Build history of the part. All positions in model axes, mm. A direction names the side the tool comes from. Round coordinates to 2 decimals unless told otherwise and drop trailing zeros. Write each loop counter-clockwise with the first axis right and the second up, starting at its lowest first coordinate (ties: lowest second). Pieces come first, ordered by that corner, then holes. Notation, with made-up numbers: (6, 38) -> (24, 38) arc R8 cw to (24, 47) -> close; hole circle Ø11 at (-25, 37). An arc over 180 degrees is marked (long way). Answer in a Markdown table with one row per item.
```python
from build123d import *

# Parameters (mm, degrees)
F0_R     = 7.8867
F1_DEPTH = 26.924
F0_R_2   = 9.144
F2_DEPTH = 2.286
F3_R     = 4.7625
F4_DEPTH = 22.225


# Not quite as in the source:
# - a length typed as a fraction of an inch, garbled in the dataset ("3 / 203.2 mm" for 3/8 in), is restored


with BuildPart() as f1:
    # F0 (on Right) → F1 (new body)
    with BuildSketch(Plane.YZ):
        Circle(F0_R)
    extrude(amount=-F1_DEPTH)

    # F0 (on Right) → F2 (join)
    with BuildSketch(Plane.YZ):
        Circle(F0_R_2)
        Circle(F0_R, mode=Mode.SUBTRACT)
        Circle(F0_R)
    extrude(amount=F2_DEPTH)

    # F3 (on face) → F4 (join)
    with BuildSketch(Plane.YZ.offset(2.286)):
        Circle(F3_R)
    extrude(amount=F4_DEPTH)


solid = f1.part
```
Q1. Saw through at C-C on x = 14.5. Write the cut outline in (y, z) (1 decimal), plus the area to 3 significant figures.
A:
| item | result |
|---|---|
| outline | circle Ø9.5 at (0, 0) |
| area | 71.3 mm² |
Q2. Drop flat-ended pins along their axis: P1, Ø10, axis at x = -7, y = 6.5, coming from the -Z side; P2, Ø8, axis at x = 14, z = 0.5, coming from the +Y side; P3, Ø3, axis at x = -10.5, y = -5.5, coming from the +Z side. Give the stop position or say it passes through.
A:
| item | result |
|---|---|
| P1 | z = -7.74 |
| P2 | y = 4.76 |
| P3 | z = 6.8 |
Q3. Saw through at D-D on z = -6. Write the cut outline in (x, y).
A:
| item | result |
|---|---|
| outline | (-26.92, -5.12) -> (0, -5.12) -> (0, -6.9) -> (2.29, -6.9) -> (2.29, 6.9) -> (0, 6.9) -> (0, 5.12) -> (-26.92, 5.12) -> close |
Q4. Saw through at A-A on y = 0. Write the cut outline in (x, z).
A:
| item | result |
|---|---|
| outline | (-26.92, -7.89) -> (0, -7.89) -> (0, -9.14) -> (2.29, -9.14) -> (2.29, -4.76) -> (24.51, -4.76) -> (24.51, 4.76) -> (2.29, 4.76) -> (2.29, 9.14) -> (0, 9.14) -> (0, 7.89) -> (-26.92, 7.89) -> close |
Q5. Which spindle directions (+Z, -Z, +X, -X, +Y, -Y) get a long thin tool onto all of the face, cutting with end or side? Do faces 1 (the flat face through (0, -7, -4)), 2 (the cylindrical face through (13.24, -3.78, -2.9)), 3 (the flat face through (24.511, 0, 0)). Say none if no direction does.
A:
| item | result |
|---|---|
| face 1 | -X |
| face 2 | +X |
| face 3 | +Z, -Z, +X, +Y, -Y |
Q6. Wall check: line 1 (X direction, y = 1, z = 7.25); line 2 (X direction, y = 0.75, z = 8.25); line 3 (Z direction, x = -10.5, y = -7.25). Give the ranges that are in metal, low to high. Write a range as [from, to].
A:
| item | result |
|---|---|
| line 1 | [-26.92, 2.29] |
| line 2 | [0, 2.29] |
| line 3 | [-3.1, 3.1] |
